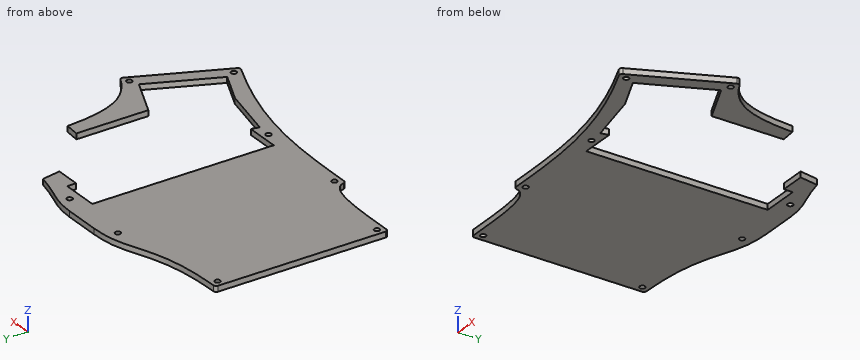
```python
from build123d import *

# Parameters (mm, degrees)
PAD007_DEPTH    = 3
POCKET010_DEPTH = 5
SKETCH042_R     = 1.45
POCKET018_DEPTH = 16
POCKET024_DEPTH = 19
FILLET005_R     = 1.5


with BuildPart() as part:
    # Sketch029 → Pad007 (new body)
    with BuildSketch(Plane.XY):
        with BuildLine():
            Line((85.725, 98.4875), (66.675, 98.4875))
            add(Edge.make_bspline(
                [(-8, 84.2), (39.625, 84.2), (39.625, 98.4875), (66.675, 98.4875)],
                knots=[0, 0, 0, 0, 1, 1, 1, 1], degree=3))
            Line((-8, 84.2), (-8, -8))
            add(Edge.make_bspline(
                [(39.625, -17.525), (39.625, -8), (20.575, -8), (-8, -8)],
                knots=[0, 0, 0, 0, 1, 1, 1, 1], degree=3))
            add(Edge.make_bspline(
                [(153.231854, -38.154949), (107.082107, -17.525), (76.2, -17.525), (39.625, -17.525)],
                knots=[0, 0, 0, 0, 1, 1, 1, 1], degree=3))
            Line((153.231854, -38.154949), (175.310198, 11.234895))
            add(Edge.make_bspline(
                [(150.875, 88.9625), (150.875, 42.8625), (150.875, 22.157965), (175.310198, 11.234895)],
                knots=[0, 0, 0, 0, 1, 1, 1, 1], degree=3))
            add(Edge.make_bspline(
                [(85.725, 98.4875), (104.775, 98.4875), (104.775, 88.9625), (150.875, 88.9625)],
                knots=[0, 0, 0, 0, 1, 1, 1, 1], degree=3))
        make_face()
    extrude(amount=PAD007_DEPTH)

    # Sketch028 → Pocket010 (cut)
    with BuildSketch(Plane(origin=(0, 0, 0), x_dir=(1, 0, 0), z_dir=(0, 0, -1))):
        Polygon((85.725, -86.475), (105.525, -86.475), (105.525, -81.7125), (143.625, -81.7125), (143.625, -17.457464), (165.732668, -7.574851), (149.57181, 28.577419), (131.568158, 20.529392), (102.96164, 14.448889), (103.848827, 10.275), (85.725, 10.275), align=None)
    extrude(amount=-POCKET010_DEPTH, mode=Mode.SUBTRACT)

    # Sketch042 → Pocket018 (cut)
    with BuildSketch(Plane.XY):
        with Locations((-4.375, -4.375)):
            Circle(SKETCH042_R)
        with Locations((-4.375, 80.575)):
            Circle(SKETCH042_R)
        with Locations((151.401832, -33.366184)):
            Circle(SKETCH042_R)
        with Locations((170.521433, 9.404873)):
            Circle(SKETCH042_R)
        with Locations((147.25, 85.3375)):
            Circle(SKETCH042_R)
        with Locations((43.25, -13.9)):
            Circle(SKETCH042_R)
        with Locations((57.15, 92.085)):
            Circle(SKETCH042_R)
        with Locations((95.25, 92.085)):
            Circle(SKETCH042_R)
        with Locations((95.25, -13.9)):
            Circle(SKETCH042_R)
    extrude(amount=POCKET018_DEPTH, mode=Mode.SUBTRACT)

    # Sketch050 → Pocket024 (cut)
    with BuildSketch(Plane.XY):
        Polygon((118.825, 80.9625), (116.825, 92.9625), (166.907578, 98.346489), (154.875, 54.9125), (142.875, 55.9125), align=None)
    extrude(amount=POCKET024_DEPTH, mode=Mode.SUBTRACT)

    # Fillet005
    fillet005_edges = [part.edges().sort_by_distance(p)[0] for p in [
        (-8, 84.2, 1.5),
        (-8, -8, 1.5),
        (39.625, -17.525, 1.5),
        (153.231854, -38.154949, 1.5),
        (175.310198, 11.234895, 1.5),
    ]]
    fillet(fillet005_edges, radius=FILLET005_R)


with BuildPart() as part_1:
    # Body006 placement: moved
    add(part.part.moved(Location((0, 0, -9))))


solid = part_1.part
```
Here's how the part is built. I have some questions about the finished solid (model axes, mm). Coordinates: 2 decimals unless noted, no trailing zeros. Loops run counter-clockwise (first coordinate to the right, second up) from the corner with the lowest first, then second, coordinate; pieces in that order, holes last. Notation, with made-up numbers: (-18.75, -14) -> (22.25, -14) arc R21 cw to (22.25, 12) -> close; hole circle Ø7 at (48.5, 86.25). An arc over 180 degrees is marked (long way). Return JSON: item names as keys, results as strings.
1) Will these pins go through, and if not, where does the flat tip stop? pin 1 (2.5 mm diameter, centred on x = 57.15, y = 92.085, fed in from +Z); pin 2 (1.5 mm diameter, centred on x = 116.5, z = -8.5, fed in from -Y); pin 3 (1.5 mm diameter, centred on x = 26.5, z = -7.5, fed in from -Y); pin 4 (0.9 mm diameter, centred on x = 90.5, z = -7.5, fed in from +Y).
Results below:
{"pin 1": "through", "pin 2": "y = -25.13", "pin 3": "y = -9.3", "pin 4": "y = 98.31"}
2) I need wall thicknesses on line 1 (Y direction, x = 43.25, z = -6.85); line 2 (X direction, y = -13.9, z = -7.6); line 3 (X direction, y = 8.5, z = -7.25) (3 decimals). Which ranges of each line are inside material? Lowest first, please. Write a range as from..to.
Results below:
{"line 1": "-17.53..-15.35, -12.45..93.78", "line 2": "38.41..41.8, 44.7..93.8, 96.7..103.08, 156.13..164.07", "line 3": "-8..85.725, 163.663..169.388, 171.654..174.088"}
3) If we section it at A-A, the plane y = 3: Write out the boundary of the cut face in (x, z) (3 decimals), then the cut area to 3 significant figures.
Results below:
{"outline": "(-8, -9) -> (85.725, -9) -> (85.725, -6) -> (-8, -6) -> close; (163.688, -9) -> (171.629, -9) -> (171.629, -6) -> (163.688, -6) -> close", "area": "305 mm²"}
4) If we section it at B-B, the plane z = -7.2: Count the separate pieces of the cut face and the enclosed holes in it, then the cut area to 3 significant figures.
Results below:
{"separate pieces": "1", "enclosed holes": "8", "area": "11,700 mm²"}
